Geometry check sheet. Reference: drawing and pictorial views, mm from the part's lowest x, y, z. A direction names the side the tool comes from. Give positions to 0.01 mm unless a question says otherwise; leave off trailing zeros. Loops run counter-clockwise (first coordinate to the right, second up) from the corner with the lowest first, then second, coordinate; pieces in that order, holes last. Notation, with made-up numbers: (76, 3) - (99, 3) arc R19 ccw to (99, 27) - close; hole circle Ø1 at (29, 39.25). An arc over 180 degrees is marked (long way). One line per question, with ' | ' between items. Start each with the question number.
1. Section check D-D, the plane z = 22.85. Enter the section's corners in (x, y), then the cut area to 3 significant figures.
2. Tool access check on the marked faces 1 and 2. Record the directions out of +Z, -Z, +X, -X, +Y, -Y that give a thin tool (end or side, any length) a straight path to the whole face; none if there is none.
3. Section check A-A, the plane x = 21.18. Enter the section's corners in (y, z), then the cut area to 3 significant figures.
4. Depth check by flat-ended pin: pin 1 Ø17.5 at (x, z) = (18, 76.5) entering from -Y; pin 2 Ø8 at (x, z) = (19.5, 21) entering from -Y. Enter the tip coordinate at first touch or a pass-through.
5. Section check B-B, the plane z = 55. Enter the section's corners in (x, y).
6. Thickness scan on line 1 along Z through (x, y) = (21, 26); line 2 along X through (y, z) = (21, 22.85); line 3 along Z through (x, y) = (110.58, 4.5). Record the ranges inside material, lowest first. Write a range as from..to.
7. Mould release check, pull along Z, two halves, no side actions. Record for the marked faces 3, 4 and 5: +Z half, -Z half, draft (parallel to the pull), parting line (faces both ways), or undercut.
8. Section check C-C, the plane y = 18. Enter the section's corners in (x, z), then the cut area to 3 significant figures.
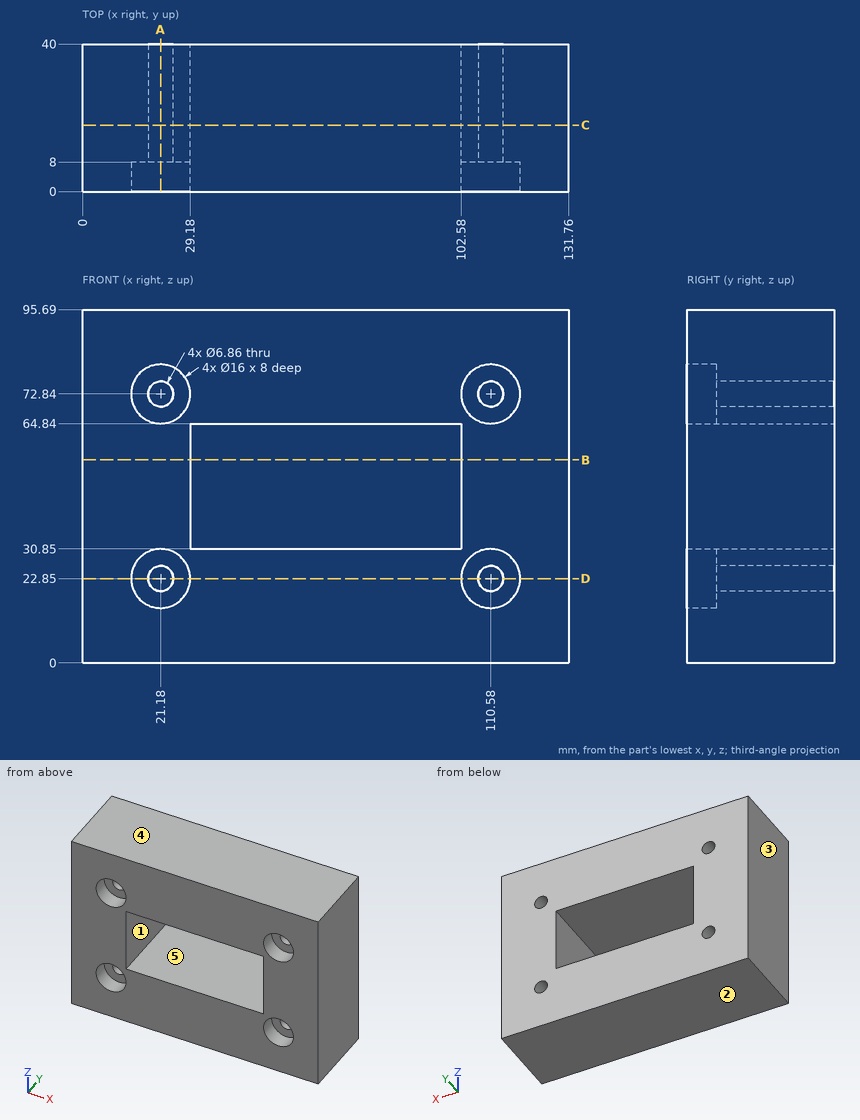
Results list:
1) outline: (0, 0) - (13.18, 0) - (13.18, 8) - (17.75, 8) - (17.75, 40) - (0, 40) - close; (24.61, 8) - (29.18, 8) - (29.18, 0) - (102.58, 0) - (102.58, 8) - (107.15, 8) - (107.15, 40) - (24.61, 40) - close; (114.01, 8) - (118.58, 8) - (118.58, 0) - (131.76, 0) - (131.76, 40) - (114.01, 40) - close | area: 4,580 mm²
2) face 1: +Y, -Y | face 2: -Z, +X, -X, +Y, -Y
3) outline: (0, 0) - (40, 0) - (40, 19.42) - (8, 19.42) - (8, 14.85) - (0, 14.85) - close; (0, 30.85) - (8, 30.85) - (8, 26.28) - (40, 26.28) - (40, 69.41) - (8, 69.41) - (8, 64.84) - (0, 64.84) - close; (0, 80.84) - (8, 80.84) - (8, 76.27) - (40, 76.27) - (40, 95.69) - (0, 95.69) - close | area: 3,130 mm²
4) pin 1: y = 0 | pin 2: y = 8
5) outline: (0, 0) - (29.18, 0) - (29.18, 40) - (0, 40) - close; (102.58, 0) - (131.76, 0) - (131.76, 40) - (102.58, 40) - close
6) line 1: 0..19.42, 26.28..69.41, 76.27..95.69 | line 2: 0..17.75, 24.61..107.15, 114.01..131.76 | line 3: 0..14.85, 30.85..64.84, 80.84..95.69
7) face 3: draft | face 4: +Z half | face 5: undercut
8) outline: (0, 0) - (131.76, 0) - (131.76, 95.69) - (0, 95.69) - close; hole circle Ø6.86 at (21.18, 22.85); hole circle Ø6.86 at (21.18, 72.84); hole (29.18, 30.85) - (102.58, 30.85) - (102.58, 64.84) - (29.18, 64.84) - close; hole circle Ø6.86 at (110.58, 22.85); hole circle Ø6.86 at (110.58, 72.84) | area: 9,970 mm²
